Autodesk Inventor part; units mm, degrees
ref_plane "YZ Plane" through (0, 0, 0) normal (1, 0, 0) x (0, 1, 0)
ref_plane "XZ Plane" through (0, 0, 0) normal (0, 1, 0) x (-1, 0, 0)
ref_plane "XY Plane" through (0, 0, 0) normal (0, 0, 1) x (1, 0, 0)
sketch "Sketch1" plane through (0, 0, 0) normal (0, 0, 1) x (1, 0, 0)
  line L0 (22.7313, 23.816) -> (22.7313, -11.184)
  line L1 (22.7313, -11.184) -> (57.7313, -11.184)
  line L2 (57.7313, -11.184) -> (57.7313, 23.816)
  line L3 (17.7313, 23.816) -> (17.7313, -16.184)
  line L4 (17.7313, -16.184) -> (62.7313, -16.184)
  line L5 (62.7313, -16.184) -> (62.7313, 23.816)
  line L6 (17.7313, 23.816) -> (22.7313, 23.816)
  line L7 (57.7313, 23.816) -> (62.7313, 23.816)
  line L8 (17.7313, 23.816) -> (62.7313, 23.816)
  point P0 (0, 0)
  point P1 (57.7313, 23.816)
  dimension "d0" = 35
  dimension "d1" = 35
  dimension "d2" = 35
  dimension "d3" = 5
extrude "Extrusion1" add sketch "Sketch1" along normal blind 5
extrude "Extrusion2" add sketch "Sketch1" along normal blind 50 contours L0 L1 L2 L7 L5 L4 L3 L6
sketch "Sketch2" plane through (57.7313, -11.184, 5) normal (-1, 0, 0) x (0, 0, 1)
  line L0 (0, 35) -> (0, 0)
  line L1 (0, 0) -> (0, 3)
  line L2 (0, 0) -> (45, 0)
  line L3 (0, 3) -> (45, 0)
  line L4 (45, 0) -> (0, 3)
  point P0 (-5, 11.184)
  dimension "d8" = 3
extrude "Extrusion3" add sketch "Sketch2" along normal blind 35
properties part number "outstorage"
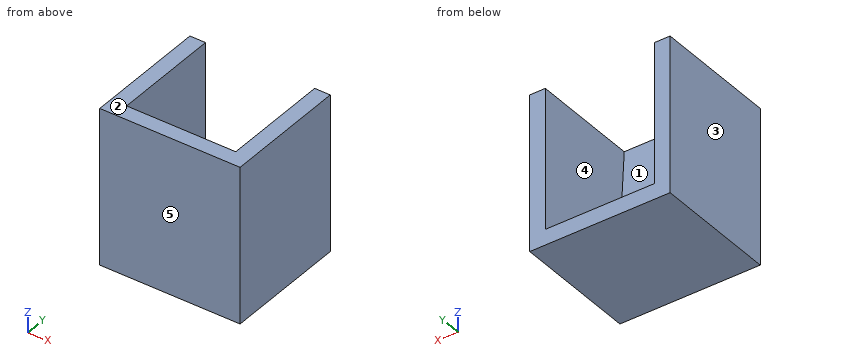
Read the model definition and answer for the solid it produces. Units are mm, in the model's axes. Face numbers are marked on the shaded views. A direction names the side the tool comes from. Coordinates: 2 decimals unless noted, no trailing zeros. Loops run counter-clockwise (first coordinate to the right, second up) from the corner with the lowest first, then second, coordinate; pieces in that order, holes last. Notation, with made-up numbers: (31, 55) -> (81, 55) arc R18 cw to (81, 77) -> close; hole circle Ø10 at (31.25, -8). An arc over 180 degrees is marked (long way). Write item = value, one per line. Start each with the question number.
1) The part is cut by section B-B, the plane z = 14. Determine the outline of the cut face in (x, y).
2) For the marked faces 1 and 2, determine the directions among +Z, -Z, +X, -X, +Y, -Y from which every point of the face is accessible in a straight line to the end or side of a thin tool.
3) The part is cut by section A-A, the plane x = 28. Determine the outline of the cut face in (y, z), plus the area to 4 significant figures.
4) Given P1, Ø16, axis at x = 33, y = 9.5, coming from the +Z side; P2, Ø1.5, axis at x = 53.5, z = 14.5, coming from the +Y side, each flat-ended and moving along its own axis, determine where each tip first touches the part or whether it passes through.
5) Find the intervals of material crossed by L1, parallel to X at y = 0.5, z = 8; L2, parallel to Z at x = 28.5, y = -4.5; L3, parallel to Y at x = 54, z = 10, in increasing order. Write a range as from..to.
6) The mould has two halves that part along X. Classify the marked faces 3, 4 and 5: pulls with the +X half, pulls with the -X half, needs draft (parallel to the pull), parting line crosses it, or undercut.
7) The part is cut by section C-C, the plane y = 3. Determine the outline of the cut face in (x, z).
Result:
q1.outline = (17.73, -16.18) -> (62.73, -16.18) -> (62.73, 23.82) -> (57.73, 23.82) -> (57.73, -8.78) -> (22.73, -8.78) -> (22.73, 23.82) -> (17.73, 23.82) -> close
q2.face_1 = +Z, +Y
q2.face_2 = +Z, +X, -X, +Y, -Y
q3.outline = (-16.18, 0) -> (23.82, 0) -> (23.82, 5) -> (-8.18, 5) -> (-11.18, 50) -> (-16.18, 50) -> close
q3.area = 492.5 mm²
q4.P1 = 5
q4.P2 = -8.77
q5.L1 = 17.73..22.73, 57.73..62.73
q5.L2 = 0..5
q5.L3 = -16.18..-8.52
q6.face_3 = pulls with the -X half
q6.face_4 = undercut
q6.face_5 = needs draft
q7.outline = (17.73, 0) -> (62.73, 0) -> (62.73, 50) -> (57.73, 50) -> (57.73, 5) -> (22.73, 5) -> (22.73, 50) -> (17.73, 50) -> close
